from build123d import *

# Parameters (mm, degrees)
SKETCH_1_W          = 15
SKETCH_1_H          = 23
EXTRUDE_1_DEPTH     = 46
SHELL_1_T           = 1.5
SKETCH_2_R          = 6
CUT_EXTRUDE_4_DEPTH = 1.5
SKETCH_3_R          = 8.25
CUT_EXTRUDE_5_DEPTH = 1.5
FILLET_2_R          = 1


with BuildPart() as part:
    # 草图1 → 凸台-拉伸1 (new body)
    with BuildSketch(Plane(origin=(0, 0, 0), x_dir=(1, 0, 0), z_dir=(0, 1, 0))):
        Rectangle(SKETCH_1_W, SKETCH_1_H)
    extrude(amount=EXTRUDE_1_DEPTH)

    # 抽壳1
    shell_1_openings = [part.faces().sort_by_distance(p)[0] for p in [
        (7.5, 23, 0),
    ]]
    offset(amount=SHELL_1_T, openings=shell_1_openings, kind=Kind.INTERSECTION)

    # 草图2 → 切除-拉伸4 (cut)
    with BuildSketch(Plane(origin=(0, 0, 0), x_dir=(-1, 0, 0), z_dir=(0, -1, 0))):
        with Locations(Location((0, 0, 0), (0, 0, 90))):
            Circle(SKETCH_2_R)
    extrude(amount=CUT_EXTRUDE_4_DEPTH, mode=Mode.SUBTRACT)

    # 草图3 → 切除-拉伸5 (cut)
    with BuildSketch(Plane.ZY.offset(9)):
        with Locations((0, 36.25)):
            Circle(SKETCH_3_R)
        with Locations(Location((0, 9.75, 0), (0, 0, 180))):
            Circle(SKETCH_3_R)
    extrude(amount=-CUT_EXTRUDE_5_DEPTH, mode=Mode.SUBTRACT)

    # 圆角2
    fillet_2_edges = [part.edges().sort_by_distance(p)[0] for p in [
        (-0.75, 47.5, -13),
        (-9, 47.5, 0),
        (-0.75, -1.5, -13),
        (-0.75, -1.5, 13),
        (-9, -1.5, 0),
        (-9, 23, -13),
        (-9, 23, 13),
        (-0.75, 47.5, 13),
    ]]
    fillet(fillet_2_edges, radius=FILLET_2_R)


solid = part.part
Geometry: final body of the model. Coordinates: model frame, mm. A direction names the side the tool comes from. Coordinates: 2 decimals unless noted, no trailing zeros. Loops run counter-clockwise (first coordinate to the right, second up) from the corner with the lowest first, then second, coordinate; pieces in that order, holes last. Notation, with made-up numbers: M -3,16.5 L 25,16.5 A18 cw 25,30.5 Z; hole C -3,51.25 d5. An arc over 180 degrees is marked long. One line per item, written item: value. Start each with the question number.
1) Cut plane C-C (x = 0). Return loops of the section in (y, z), then the cut area to 3 significant figures.
2) Material intervals for L1, parallel to Y at x = -7.8, z = 0; L2, parallel to Y at x = 1.5, z = -10.5; L3, parallel to Y at x = -8.5, z = 0, sorted ascending. Write a range as from..to.
3) Draft query along Z for faces 4 (the cylindrical face through (-8.715, 22.671, -12.699)), 5 (the flat face through (0, 23, 11.5)), 6 (the cylindrical face through (-8.715, -1.199, -0.168)). Return one class per face: released by +Z, released by -Z, zero draft, split by the parting line, or undercut.
4) Reachability of faces 1 (the flat face through (-3.4, 0, -5.3)), 2 (the cylindrical face through (1.802, -0.74, -5.723)), 3 (the flat face through (7.5, 23, 12)) from +Z, -Z, +X, -X, +Y, -Y: full face, straight path, thin tool, end or side. Return the list, or none.
5) Cut plane B-B (y = 36.25). Return loops of the section in (x, z).
6) Cut plane A-A (z = 0). Return loops of the section in (x, y).
7) Pin query (flat end, axial travel): P1, Ø2, axis at y = 27.5, z = -5, coming from the +X side; P2, Ø10, axis at y = 9.75, z = 0, coming from the +X side (3 decimals); P3, Ø7, axis at x = 0, z = 0, coming from the -Y side. Return the tip coordinate at first contact, or that it passes through.
8) Cut plane D-D (x = 6.75). Return loops of the section in (y, z), then the cut area to 3 significant figures.
Evaluation:
1. outline: M -1.5,-12 A1 ccw -0.5,-13 L 46.5,-13 A1 ccw 47.5,-12 L 47.5,12 A1 ccw 46.5,13 L -0.5,13 A1 ccw -1.5,12 L -1.5,6 L 0,6 L 0,11.5 L 46,11.5 L 46,-11.5 L 0,-11.5 L 0,-6 L -1.5,-6 Z
1. area: 197 mm^2
2. L1: -1.5..1.5, 18..28, 44.5..47.5
2. L2: -1.5..0, 46..47.5
2. L3: -1.37..1.5, 18..28, 44.5..47.37
3. face 4: released by -Z
3. face 5: undercut
3. face 6: zero draft
4. face 1: +X
4. face 2: -Y
4. face 3: +Z, -Z, +X, +Y, -Y
5. outline: M -9,-12 A1 ccw -8,-13 L 7.5,-13 L 7.5,-11.5 L -7.5,-11.5 L -7.5,-8.25 L -9,-8.25 Z; M -9,8.25 L -7.5,8.25 L -7.5,11.5 L 7.5,11.5 L 7.5,13 L -8,13 A1 ccw -9,12 Z
6. outline: M -9,-0.5 A1 ccw -8,-1.5 L -6,-1.5 L -6,0 L -7.5,0 L -7.5,1.5 L -9,1.5 Z; M -9,18 L -7.5,18 L -7.5,28 L -9,28 Z; M -9,44.5 L -7.5,44.5 L -7.5,46 L 7.5,46 L 7.5,47.5 L -8,47.5 A1 ccw -9,46.5 Z; M 6,-1.5 L 7.5,-1.5 L 7.5,0 L 6,0 Z
7. P1: x = -7.5
7. P2: through
7. P3: y = 46
8. outline: M -1.5,-12 A1 ccw -0.5,-13 L 46.5,-13 A1 ccw 47.5,-12 L 47.5,12 A1 ccw 46.5,13 L -0.5,13 A1 ccw -1.5,12 Z; hole M 0,-11.5 L 46,-11.5 L 46,11.5 L 0,11.5 Z
8. area: 215 mm^2
